from build123d import *

# Parameters (mm, degrees)
F_3_48_TAPPED_HOLE1_D = 1.9939
CIRPATTERN1_COUNT     = 12
BOSS_EXTRUDE1_DEPTH   = 3.175


with BuildPart() as part:
    # Cross Section → Main (revolve)
    with BuildSketch(Plane.XY):
        with BuildLine():
            Line((-38.1, 0), (-38.1, -3.175))
            Line((-38.1, -3.175), (-41.2242, -3.175))
            Line((-41.2242, -3.175), (-41.2242, -15.875))
            Line((-41.2242, -15.875), (-44.3992, -15.875))
            Line((-44.3992, -15.875), (-44.3992, -3.175))
            Line((-44.3992, -3.175), (-51.2572, -3.175))
            Line((-51.2572, -3.175), (-51.2572, 9.525))
            Line((-51.2572, 9.525), (-49.784, 9.525))
            Line((-49.784, 9.525), (-49.784, 1.5875))
            Line((-49.784, 1.5875), (-39.6875, 1.5875))
            ThreePointArc((-39.6875, 1.5875), (-38.564967985, 1.122532015), (-38.1, 0))
        make_face()
    revolve(axis=Axis((0, 55, 0), (0, -1, 0)))

    # #3-48 Tapped Hole1 (through all)
    with Locations(Plane(origin=(0, 1.5875, 0), x_dir=(1, 0, 0), z_dir=(0, 1, 0))):
        with Locations((-45.5549, 0)):
            f_3_48_tapped_hole1 = Hole(F_3_48_TAPPED_HOLE1_D / 2)

    # CirPattern1: #3-48 Tapped Hole1 ×12 about axis
    cirpattern1_axis = Axis((0, 0, 0), (0, 1, 0))
    for i in range(1, CIRPATTERN1_COUNT):
        add(f_3_48_tapped_hole1.rotate(cirpattern1_axis, i * 360 / CIRPATTERN1_COUNT), mode=Mode.SUBTRACT)

    # Sketch3 → Boss-Extrude1 (add)
    with BuildSketch(Plane(origin=(0, 1.5875, 0), x_dir=(1, 0, 0), z_dir=(0, 1, 0))):
        with BuildLine():
            Line((-47.168007396, -15.925631363), (-42.677879335, -11.435503303))
            Line((-42.677879335, -11.435503303), (-48.811508332, -9.792002366))
            ThreePointArc((-48.811508332, -9.792002366), (-48.087651336, -12.885047341), (-47.168007396, -15.925631363))
        make_face()
    extrude(amount=BOSS_EXTRUDE1_DEPTH)


solid = part.part
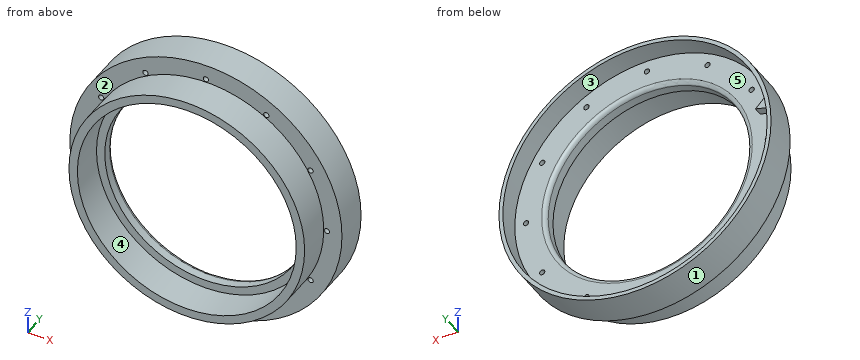
Geometry check sheet. Reference: the model listing, model coordinates, mm. Face numbers are marked on the shaded views. A direction names the side the tool comes from. Give positions to 0.01 mm unless a question says otherwise; leave off trailing zeros. Loops run counter-clockwise (first coordinate to the right, second up) from the corner with the lowest first, then second, coordinate; pieces in that order, holes last. Notation, with made-up numbers: (82.5, 84) -> (117.5, 84) arc R12 cw to (117.5, 93) -> close; hole circle Ø10 at (75.25, -3). An arc over 180 degrees is marked (long way). Answer in a Markdown table with one row per item. Add a question column.
1) Cross-section at A-A on y = -7. Record the boundary of the cut face in (x, z), and give its area (3 significant figures).
2) Set-up check for the marked faces 4 and 5: record each of +Z, -Z, +X, -X, +Y, -Y from which the full face is reachable in a straight line by a thin tool's end or side.
3) Draft check along X on the marked faces 1, 2 and 3. Enter one of: pulls with the +X half, pulls with the -X half, needs draft (parallel to the pull), parting line crosses it, or undercut.
4) Gauge pin test, flat ends, axial feed: P1, Ø3, axis at x = -45.55, z = 0, coming from the +Y side; P2, Ø12, axis at x = -15, z = -29.5, coming from the +Y side; P3, Ø1, axis at y = -10, z = 36, coming from the +X side. Record the tip position at first contact, or that the pin passes through.
5) Material ranges on probe 1 along Y at (x, z) = (-43, 15) (1 decimal); probe 2 along X at (y, z) = (5.25, 0); probe 3 along Z at (x, y) = (30, -9), recorded low to high. Write a range as from..to.
Outcome:
| question | item | result |
|---|---|---|
| 1 | outline | circle Ø88.8 at (0, 0); hole circle Ø82.45 at (0, 0) |
| 1 | area | 854 mm^2 |
| 2 | face 4 | -Y |
| 2 | face 5 | +Y |
| 3 | face 1 | parting line crosses it |
| 3 | face 2 | needs draft |
| 3 | face 3 | undercut |
| 4 | P1 | stops at y = 1.59 |
| 4 | P2 | stops at y = 1.47 |
| 4 | P3 | stops at x = 26.67 |
| 5 | probe 1 | y = -3.2..1.6 |
| 5 | probe 2 | x = -51.26..-49.78, 49.78..51.26 |
| 5 | probe 3 | z = -32.73..-28.27, 28.27..32.73 |
